from build123d import *

# Parameters (mm, degrees)
SKETCH1_W           = 51
SKETCH1_H           = 82
SKETCH1_R           = 1.6
BOSS_EXTRUDE1_DEPTH = 25
SKETCH1_3_W         = 10
SKETCH1_3_H         = 8.5
SKETCH1_3_H_2       = 26
BOSS_EXTRUDE2_DEPTH = 10
FILLET1_R           = 5


with BuildPart() as part:
    # Sketch1 → Boss-Extrude1 (new body)
    with BuildSketch(Plane(origin=(0, 0, 0), x_dir=(1, 0, 0), z_dir=(0, 1, 0))):
        Rectangle(SKETCH1_W, SKETCH1_H)
        with Locations(Location((0, -37.1, 0), (0, 0, 270))):
            Circle(SKETCH1_R, mode=Mode.SUBTRACT)
        with Locations(Location((0, 37.1, 0), (0, 0, 270))):
            Circle(SKETCH1_R, mode=Mode.SUBTRACT)
    extrude(amount=BOSS_EXTRUDE1_DEPTH)

    # Sketch1_3 → Boss-Extrude2 (add)
    with BuildSketch(Plane(origin=(0, 0, 0), x_dir=(1, 0, 0), z_dir=(0, 1, 0))):
        with Locations((30.5, -21.25)):
            Rectangle(SKETCH1_3_W, SKETCH1_3_H)
        with Locations((-30.5, -18)):
            Rectangle(SKETCH1_3_W, SKETCH1_3_H_2)
    extrude(amount=BOSS_EXTRUDE2_DEPTH)

    # Fillet1
    fillet1_edges = [part.edges().sort_by_distance(p)[0] for p in [
        (-25.5, 12.5, 41),
        (-25.5, 12.5, -41),
        (25.5, 12.5, -41),
        (25.5, 12.5, 41),
    ]]
    fillet(fillet1_edges, radius=FILLET1_R)


solid = part.part
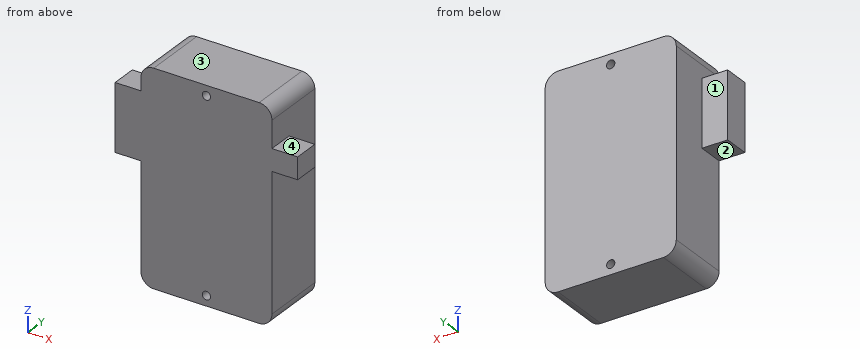
Can you work these out from the model? Positions are in its coordinate system, mm. Face numbers are marked on the shaded views. A direction names the side the tool comes from. Coordinates: 2 decimals unless noted, no trailing zeros. Loops run counter-clockwise (first coordinate to the right, second up) from the corner with the lowest first, then second, coordinate; pieces in that order, holes last. Notation, with made-up numbers: (-34.75, 67) - (22.25, 67) arc R6 cw to (22.25, 77) - close; hole circle Ø8 at (80.25, 4.25). An arc over 180 degrees is marked (long way). Answer as a JSON object with one key per item and string values. Group by question number.
Item 1: If I drill on L1, parallel to X at y = 6.25, z = 10.5; L2, parallel to X at y = 21.25, z = -1.5; L3, parallel to Z at x = -27, y = 2, over which ranges is the centre line in solid material (lowest first)? Write a range as from..to.
Item 2: If we section it at C-C (z = -37.1): List the corners of the cut face in (x, y) for me.
Item 3: If we section it at D-D (z = 22.5): List the corners of the cut face in (x, y) for me, plus the area to 4 significant figures.
Item 4: On a 3-axis mill with a long thin cutter (end or side, diameter ignored), from which of +Z, -Z, +X, -X, +Y, -Y can I reach the whole of each face in a straight line? I mean the marked faces 1, 2, 3 and 4. Say none if no direction works.
Item 5: For pin 1 (3 mm diameter, centred on x = -28.5, y = 2.5, fed in from -Z); pin 2 (1 mm diameter, centred on y = 7.5, z = -10.5, fed in from +X); pin 3 (1.5 mm diameter, centred on y = 14.5, z = 27.5, fed in from -X), each with a flat end and sliding along its axis, tell me the tip position at first contact or that it passes through.
Item 6: If we section it at B-B (y = 6): List the corners of the cut face in (x, z) for me.
Item 7: If we section it at A-A (x = 0): List the corners of the cut face in (y, z) for me.
Returned:
{
 "1": {"L1": "x = -35.5..25.5", "L2": "x = -25.5..25.5", "L3": "z = 5..31"},
 "2": {"outline": "(-25.38, 0) - (-1.6, 0) - (-1.6, 25) - (-25.38, 25) - close; (1.6, 0) - (25.38, 0) - (25.38, 25) - (1.6, 25) - close"},
 "3": {"outline": "(-35.5, 0) - (35.5, 0) - (35.5, 10) - (25.5, 10) - (25.5, 25) - (-25.5, 25) - (-25.5, 10) - (-35.5, 10) - close", "area": "1,475 mm²"},
 "4": {"face 1": "+Z, -Z, -X, +Y", "face 2": "-Z, -X, +Y, -Y", "face 3": "+Z, +X, -X, +Y, -Y", "face 4": "+Z, +X, +Y, -Y"},
 "5": {"pin 1": "stops at z = 5", "pin 2": "stops at x = 25.5", "pin 3": "stops at x = -25.5"},
 "6": {"outline": "(-35.5, 5) - (-25.5, 5) - (-25.5, -36) arc R5 ccw to (-20.5, -41) - (20.5, -41) arc R5 ccw to (25.5, -36) - (25.5, 17) - (35.5, 17) - (35.5, 25.5) - (25.5, 25.5) - (25.5, 36) arc R5 ccw to (20.5, 41) - (-20.5, 41) arc R5 ccw to (-25.5, 36) - (-25.5, 31) - (-35.5, 31) - close; hole circle Ø3.2 at (0, -37.1); hole circle Ø3.2 at (0, 37.1)"},
 "7": {"outline": "(0, -41) - (25, -41) - (25, -38.7) - (0, -38.7) - close; (0, -35.5) - (25, -35.5) - (25, 35.5) - (0, 35.5) - close; (0, 38.7) - (25, 38.7) - (25, 41) - (0, 41) - close"}
}
